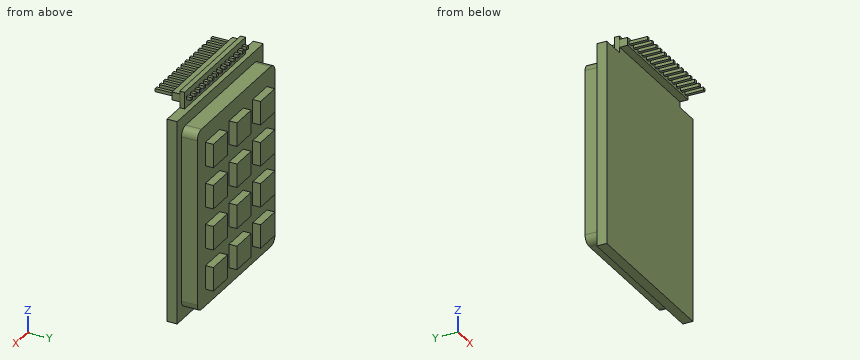
from build123d import *

# Parameters (mm, degrees)
ESQUISSE1_W             = 51
ESQUISSE1_H             = 64
BOSS_EXTRU_1_DEPTH      = 3.15
BOSS_EXTRU_2_DEPTH      = 5
ESQUISSE3_W             = 8.4
ESQUISSE3_H             = 7.45
BOSS_EXTRU_3_DEPTH      = 2.5
ESQUISSE4_W             = 36
ESQUISSE4_H             = 5.25
BOSS_EXTRU_4_DEPTH      = 1.54
ESQUISSE5_W             = 35.72
ESQUISSE5_H             = 2.5
BOSS_EXTRU_5_DEPTH      = 2.52
ESQUISSE6_W             = 1
ESQUISSE6_H             = 1
BOSS_EXTRU_6_DEPTH      = 5.75
BOSS_EXTRU_6_DEPTH_BACK = 5.52


with BuildPart() as part:
    # Esquisse1 → Boss.-Extru.1 (new body)
    with BuildSketch(Plane(origin=(0, 0, 0), x_dir=(1, 0, 0), z_dir=(0, 1, 0))):
        with Locations((25.5, 32)):
            Rectangle(ESQUISSE1_W, ESQUISSE1_H)
    extrude(amount=BOSS_EXTRU_1_DEPTH)

    # Esquisse2 → Boss.-Extru.2 (add)
    with BuildSketch(Plane(origin=(0, 3.15, 0), x_dir=(1, 0, 0), z_dir=(0, 1, 0))):
        with BuildLine():
            Line((2.5, 58), (2.5, 6))
            ThreePointArc((2.5, 6), (3.232233047, 4.232233047), (5, 3.5))
            Line((5, 3.5), (46, 3.5))
            ThreePointArc((46, 3.5), (47.767766953, 4.232233047), (48.5, 6))
            Line((48.5, 6), (48.5, 58))
            ThreePointArc((48.5, 58), (47.767766953, 59.767766953), (46, 60.5))
            Line((46, 60.5), (5, 60.5))
            ThreePointArc((5, 60.5), (3.232233047, 59.767766953), (2.5, 58))
        make_face()
    extrude(amount=BOSS_EXTRU_2_DEPTH)

    # Esquisse3 → Boss.-Extru.3 (add)
    with BuildSketch(Plane(origin=(0, 8.15, 0), x_dir=(1, 0, 0), z_dir=(0, 1, 0))):
        with Locations((11.5, 38.5)):
            Rectangle(ESQUISSE3_W, ESQUISSE3_H)
        with Locations((11.5, 51.5)):
            Rectangle(ESQUISSE3_W, ESQUISSE3_H)
        with Locations((25.5, 51.5)):
            Rectangle(ESQUISSE3_W, ESQUISSE3_H)
        with Locations((39.5, 51.5)):
            Rectangle(ESQUISSE3_W, ESQUISSE3_H)
        with Locations((25.5, 38.5)):
            Rectangle(ESQUISSE3_W, ESQUISSE3_H)
        with Locations((39.5, 38.5)):
            Rectangle(ESQUISSE3_W, ESQUISSE3_H)
        with Locations((11.5, 12.5)):
            Rectangle(ESQUISSE3_W, ESQUISSE3_H)
        with Locations((11.5, 25.5)):
            Rectangle(ESQUISSE3_W, ESQUISSE3_H)
        with Locations((25.5, 25.5)):
            Rectangle(ESQUISSE3_W, ESQUISSE3_H)
        with Locations((39.5, 25.5)):
            Rectangle(ESQUISSE3_W, ESQUISSE3_H)
        with Locations((25.5, 12.5)):
            Rectangle(ESQUISSE3_W, ESQUISSE3_H)
        with Locations((39.5, 12.5)):
            Rectangle(ESQUISSE3_W, ESQUISSE3_H)
    extrude(amount=BOSS_EXTRU_3_DEPTH)

    # Esquisse4 → Boss.-Extru.4 (add)
    with BuildSketch(Plane.XZ):
        with Locations((25.5, 2.625)):
            Rectangle(ESQUISSE4_W, ESQUISSE4_H)
    extrude(amount=-BOSS_EXTRU_4_DEPTH)

    # Esquisse5 → Boss.-Extru.5 (add)
    with BuildSketch(Plane.XZ):
        with Locations((25.5, 3)):
            Rectangle(ESQUISSE5_W, ESQUISSE5_H)
    extrude(amount=BOSS_EXTRU_5_DEPTH)

    # Esquisse6 → Boss.-Extru.6 (add, two sides)
    with BuildSketch(Plane.XZ.offset(2.52)) as boss_extru_6_sk:
        with Locations((9.041511345, 3)):
            Rectangle(ESQUISSE6_W, ESQUISSE6_H)
        with Locations((11.581511345, 3)):
            Rectangle(ESQUISSE6_W, ESQUISSE6_H)
        with Locations((14.121511345, 3)):
            Rectangle(ESQUISSE6_W, ESQUISSE6_H)
        with Locations((16.661511345, 3)):
            Rectangle(ESQUISSE6_W, ESQUISSE6_H)
        with Locations((19.201511345, 3)):
            Rectangle(ESQUISSE6_W, ESQUISSE6_H)
        with Locations((21.741511345, 3)):
            Rectangle(ESQUISSE6_W, ESQUISSE6_H)
        with Locations((24.281511345, 3)):
            Rectangle(ESQUISSE6_W, ESQUISSE6_H)
        with Locations((26.821511345, 3)):
            Rectangle(ESQUISSE6_W, ESQUISSE6_H)
        with Locations((29.361511345, 3)):
            Rectangle(ESQUISSE6_W, ESQUISSE6_H)
        with Locations((31.901511345, 3)):
            Rectangle(ESQUISSE6_W, ESQUISSE6_H)
        with Locations((34.441511345, 3)):
            Rectangle(ESQUISSE6_W, ESQUISSE6_H)
        with Locations((36.981511345, 3)):
            Rectangle(ESQUISSE6_W, ESQUISSE6_H)
        with Locations((39.521511345, 3)):
            Rectangle(ESQUISSE6_W, ESQUISSE6_H)
        with Locations((42.061511345, 3)):
            Rectangle(ESQUISSE6_W, ESQUISSE6_H)
    extrude(amount=BOSS_EXTRU_6_DEPTH)
    extrude(boss_extru_6_sk.sketch, amount=-BOSS_EXTRU_6_DEPTH_BACK)


solid = part.part
Model file for the job. Use its own axes, mm. Give positions to 0.01 mm unless a question says otherwise; leave off trailing zeros. Loops run counter-clockwise (first coordinate to the right, second up) from the corner with the lowest first, then second, coordinate; pieces in that order, holes last. Notation, with made-up numbers: (5, 44) -> (52, 44) arc R31 cw to (52, 69) -> close; hole circle Ø11 at (-1, 41.25). An arc over 180 degrees is marked (long way). Use a Markdown table: item, result. Add a question column.
(1) Wall check: line 1 along Z through (x, y) = (22, 10) (3 decimals); line 2 along Y through (x, z) = (24, -26); line 3 along Y through (x, z) = (46.5, -41). Give the ranges that are in metal, low to high.
(2) Drop flat-ended pins along their axis: pin 1 Ø0.5 at (x, y) = (27, -4.5) entering from -Z; pin 2 Ø0.8 at (x, y) = (29, -6.5) entering from +Z; pin 3 Ø1 at (x, z) = (22.5, -20.5) entering from +Y. Give the stop position or say it passes through.
(3) Slice it at A-A on z = -38.5. List the corners of the cut face in (x, y).
(4) Slice it at D-D on y = -0.75. List the corners of the cut face in (x, z).
(5) Slice it at C-C on z = -20. List the corners of the cut face in (x, y), and give its area (3 significant figures).
(6) Slice it at B-B on y = 5.25. List the corners of the cut face in (x, z).
Filled sheet:
| question | item | result |
|---|---|---|
| 1 | line 1 | -55.225 to -47.775, -42.225 to -34.775, -29.225 to -21.775, -16.225 to -8.775 |
| 1 | line 2 | 0 to 10.65 |
| 1 | line 3 | 0 to 8.15 |
| 2 | pin 1 | z = 2.5 |
| 2 | pin 2 | z = 3.5 |
| 2 | pin 3 | y = 8.15 |
| 3 | outline | (0, 0) -> (51, 0) -> (51, 3.15) -> (48.5, 3.15) -> (48.5, 8.15) -> (43.7, 8.15) -> (43.7, 10.65) -> (35.3, 10.65) -> (35.3, 8.15) -> (29.7, 8.15) -> (29.7, 10.65) -> (21.3, 10.65) -> (21.3, 8.15) -> (15.7, 8.15) -> (15.7, 10.65) -> (7.3, 10.65) -> (7.3, 8.15) -> (2.5, 8.15) -> (2.5, 3.15) -> (0, 3.15) -> close |
| 4 | outline | (7.64, 1.75) -> (43.36, 1.75) -> (43.36, 4.25) -> (7.64, 4.25) -> close |
| 5 | outline | (0, 0) -> (51, 0) -> (51, 3.15) -> (48.5, 3.15) -> (48.5, 8.15) -> (2.5, 8.15) -> (2.5, 3.15) -> (0, 3.15) -> close |
| 5 | area | 391 mm2 |
| 6 | outline | (2.5, -58) arc R2.5 ccw to (5, -60.5) -> (46, -60.5) arc R2.5 ccw to (48.5, -58) -> (48.5, -6) arc R2.5 ccw to (46, -3.5) -> (5, -3.5) arc R2.5 ccw to (2.5, -6) -> close |
